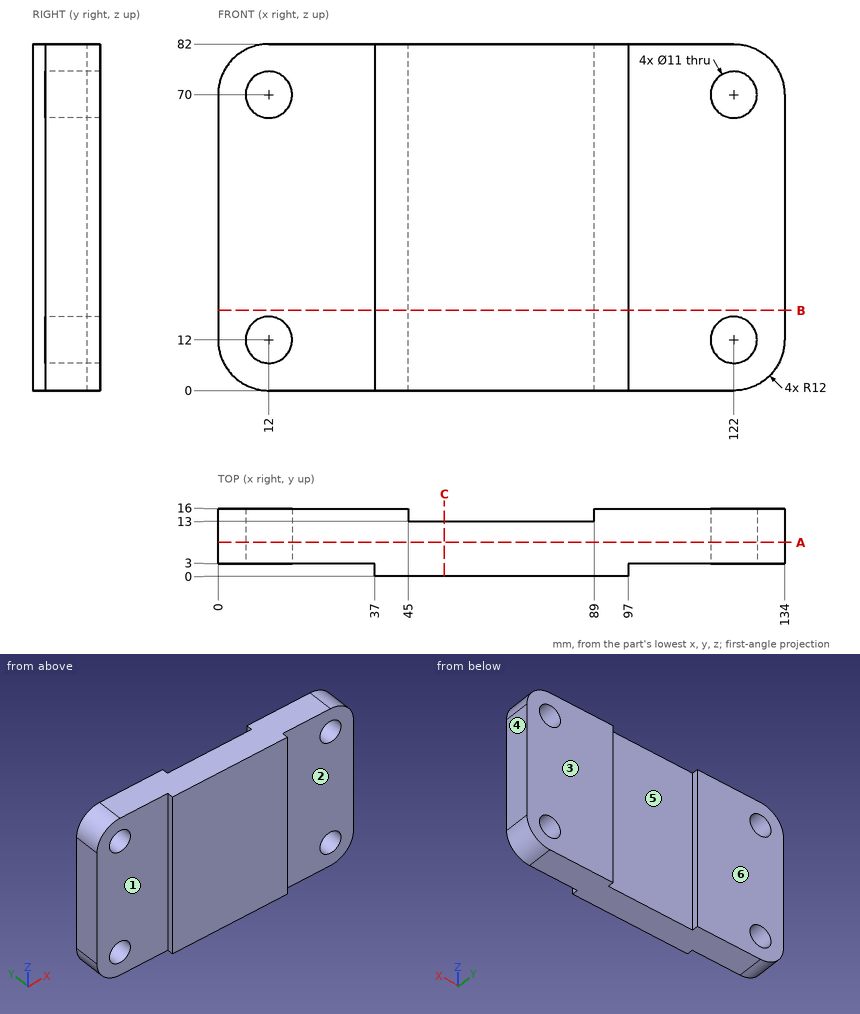
Part print with two shaded views. Sizes in mm from the minimum x, y, z corner. A direction names the side the tool comes from. Round coordinates to 2 decimals unless told otherwise and drop trailing zeros. Write each loop counter-clockwise with the first axis right and the second up, starting at its lowest first coordinate (ties: lowest second). Pieces come first, ordered by that corner, then holes. Notation, with made-up numbers: (9.25, 0) -> (58.25, 0) arc R14 cw to (58.25, 7) -> close; hole circle Ø3 at (-17, 54.5). An arc over 180 degrees is marked (long way). Put each result on its own line as item: value.
Item 1: Slice it at C-C, the plane x = 53.5. Give the cut face in (y, z), plus the area to 3 significant figures.
Here are the results:
outline: (0, 0) -> (13, 0) -> (13, 82) -> (0, 82) -> close
area: 1,070 mm^2
Item 2: Tool access for the marked faces 1, 2 and 3: list every direction of +Z, -Z, +X, -X, +Y, -Y with a clear straight run to the whole face (end or side of a thin tool).
Here are the results:
face 1: +Z, -Z, -X, -Y
face 2: +Z, -Z, +X, -Y
face 3: +Z, -Z, +X, -X, +Y
Item 3: Wall check: probe 1 along Z at (x, y) = (12, 9.5); probe 2 along X at (y, z) = (3.5, 14); probe 3 along Z at (x, y) = (9, 10.25). Give the ranges that are in metal, low to high. Write a range as from..to.
Here are the results:
probe 1: z = 0..6.5, 17.5..64.5, 75.5..82
probe 2: x = 0..6.88, 17.12..116.88, 127.12..134
probe 3: z = 0.38..7.39, 16.61..65.39, 74.61..81.62
Item 4: Slice it at A-A, the plane y = 8. Give the cut face in (x, z).
Here are the results:
outline: (0, 12) arc R12 ccw to (12, 0) -> (122, 0) arc R12 ccw to (134, 12) -> (134, 70) arc R12 ccw to (122, 82) -> (12, 82) arc R12 ccw to (0, 70) -> close; hole circle Ø11 at (12, 12); hole circle Ø11 at (12, 70); hole circle Ø11 at (122, 12); hole circle Ø11 at (122, 70)
Item 5: Slice it at B-B, the plane z = 19. Give the cut face in (x, y).
Here are the results:
outline: (0, 3) -> (37, 3) -> (37, 0) -> (97, 0) -> (97, 3) -> (134, 3) -> (134, 16) -> (89, 16) -> (89, 13) -> (45, 13) -> (45, 16) -> (0, 16) -> close
Item 6: Flat gauge pins, fed straight in: P1, Ø2, axis at x = 100.5, z = 9.5, coming from the -Y side; P2, Ø9, axis at x = 122, z = 70, coming from the +Y side; P3, Ø2.5, axis at y = 1.5, z = 22, coming from the +X side; P4, Ø5, axis at x = 80, z = 41.5, coming from the +Y side. Where does each tip first touch, or does it go through?
Here are the results:
P1: stops at y = 3
P2: passes through
P3: stops at x = 97
P4: stops at y = 13
Item 7: Two-plate mould, pull along X, no slides. Class the marked faces 4, 5 and 6: pulls with the +X half, pulls with the -X half, needs draft (parallel to the pull), parting line crosses it, or undercut.
Here are the results:
face 4: pulls with the +X half
face 5: undercut
face 6: needs draft
